from build123d import *

# Parameters (mm, degrees)
BOSS_EXTRUDE1_DEPTH = 346.86875
SKETCH2_R           = 3.2639
CUT_EXTRUDE1_DEPTH  = 12.7
SKETCH3_R           = 3.2639
CUT_EXTRUDE2_DEPTH  = 12.7


with BuildPart() as part:
    # Sketch1 → Boss-Extrude1 (new body)
    with BuildSketch(Plane(origin=(0, 0, 0), x_dir=(0, 0, -1), z_dir=(1, 0, 0))):
        Polygon((0, 7.332348419), (-6.35, 3.666174209), (-6.35, -3.666174209), (0, -7.332348419), (6.35, -3.666174209), (6.35, 3.666174209), align=None)
    extrude(amount=BOSS_EXTRUDE1_DEPTH)

    # Sketch2 → Cut-Extrude1 (cut)
    with BuildSketch(Plane(origin=(346.86875, 0, 0), x_dir=(0, 0, -1), z_dir=(1, 0, 0))):
        Circle(SKETCH2_R)
    extrude(amount=-CUT_EXTRUDE1_DEPTH, mode=Mode.SUBTRACT)

    # Sketch3 → Cut-Extrude2 (cut)
    with BuildSketch(Plane.ZY):
        Circle(SKETCH3_R)
    extrude(amount=-CUT_EXTRUDE2_DEPTH, mode=Mode.SUBTRACT)


solid = part.part
For this review, take the finished solid that the model builds, in its own axes (mm). A direction names the side the tool comes from. Give positions to 0.01 mm unless a question says otherwise; leave off trailing zeros. Loops run counter-clockwise (first coordinate to the right, second up) from the corner with the lowest first, then second, coordinate; pieces in that order, holes last. Notation, with made-up numbers: (40, 17.5) - (45, 17.5) arc R15 ccw to (45, 38.5) - close; hole circle Ø10 at (42, 12.5). An arc over 180 degrees is marked (long way). Write each question's results on one line, items separated by ' | '.
(1) Take a section at B-B (x = 108.5). Give the boundary of the cut face in (y, z).
Conclusion:
outline: (-7.33, 0) - (-3.67, -6.35) - (3.67, -6.35) - (7.33, 0) - (3.67, 6.35) - (-3.67, 6.35) - close
(2) For line 1 along Y through (x, z) = (343.25, 0); line 2 along X through (y, z) = (-1.5, 2.75); line 3 along Z through (x, y) = (80, 6.25), list the stretches that pass through material, from the lowest coordinate up.
Conclusion:
line 1: -7.33 to -3.26, 3.26 to 7.33 | line 2: 12.7 to 334.17 | line 3: -1.87 to 1.87
(3) Draft analysis for pull direction Y (two halves, no side actions). For faces 1 (the cylindrical face through (340.608, -3.186, 0.708)), 2 (the flat face through (171, 0, -6.35)), 3 (the flat face through (171.006, 5.474, -3.219)), state which applies: +Y half, -Y half, draft (parallel to the pull), parting line (faces both ways), or undercut.
Conclusion:
face 1: undercut | face 2: draft | face 3: +Y half
(4) For pin 1 Ø6 at (y, z) = (0, 0) entering from +X; pin 2 Ø1.5 at (x, y) = (111.5, 4.5) entering from +Z; pin 3 Ø2 at (y, z) = (1, 1) entering from -X, all flat-tipped, find the tip position at first contact; note any pin that passes through.
Conclusion:
pin 1: x = 334.17 | pin 2: z = 6.2 | pin 3: x = 12.7
(5) Take a section at A-A (y = 0). Give the boundary of the cut face in (x, z).
Conclusion:
outline: (0, -6.35) - (346.87, -6.35) - (346.87, -3.26) - (334.17, -3.26) - (334.17, 3.26) - (346.87, 3.26) - (346.87, 6.35) - (0, 6.35) - (0, 3.26) - (12.7, 3.26) - (12.7, -3.26) - (0, -3.26) - close
(6) For faces 4 (the flat face through (12.7, 0, 0)), 5 (the flat face through (334.169, 0, 0)), 6 (the flat face through (171.006, -5.525, -3.131)), list the 3-axis set-ups (+Z, -Z, +X, -X, +Y, -Y) from which the entire face can be reached by the end or side of a thin tool; tool diameter is ignored.
Conclusion:
face 4: -X | face 5: +X | face 6: -Z, +X, -X, -Y
